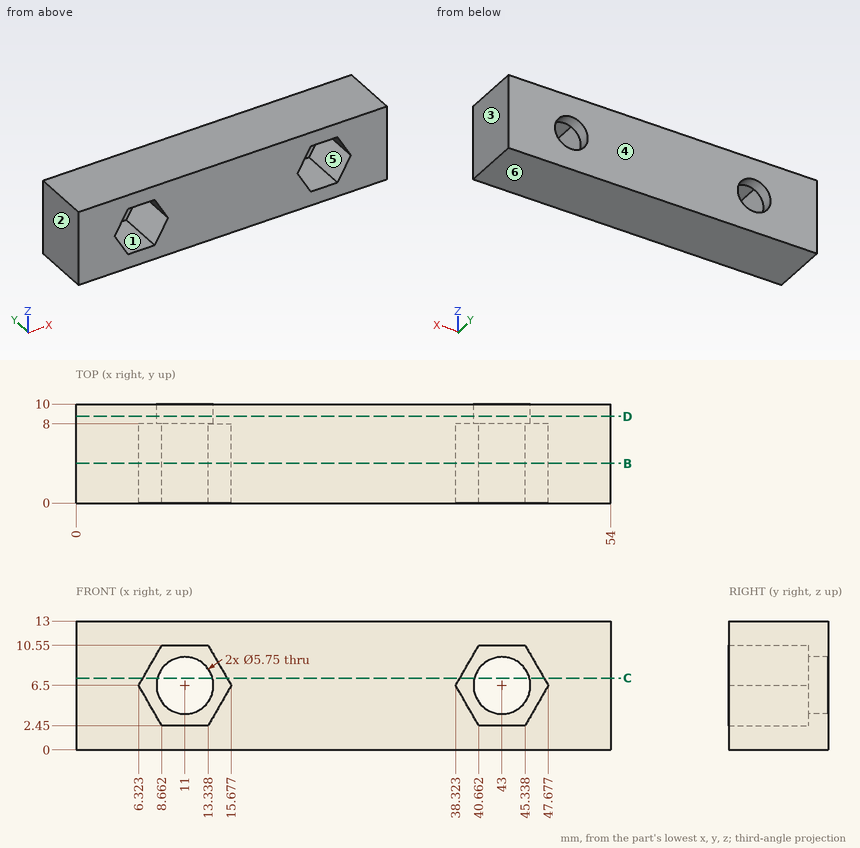
Can you work these out from the drawing? Everything is in mm from the part's minimum corner. A direction names the side the tool comes from. Give positions to 0.01 mm unless a question says otherwise; leave off trailing zeros. Write each loop counter-clockwise with the first axis right and the second up, starting at its lowest first coordinate (ties: lowest second). Pieces come first, ordered by that corner, then holes. Notation, with made-up numbers: M 46.5,6 L 85.5,6 A18 cw 85.5,12 Z; hole C 58.25,-21 d3. An arc over 180 degrees is marked long. Answer in a Markdown table with one row per item. Add a question column.
Item 1: Imagine slicing it at C-C, the plane z = 7.25. Write out the boundary of the cut face in (x, y) (1 decimal), plus the area to 3 significant figures.
Item 2: Imagine slicing it at B-B, the plane y = 4. Write out the boundary of the cut face in (x, z).
Item 3: We'd pull the mould along X, two halves only. Please class the marked faces 1, 2, 3 and 4: released by +X, released by -X, zero draft, split by the parting line, or undercut.
Item 4: Please list where these lines run through material, in increasing order: L1, parallel to Z at x = 43, y = 9.35 (1 decimal); L2, parallel to X at y = 4, z = 7.5; L3, parallel to X at y = 1, z = 6.75.
Item 5: Imagine slicing it at D-D, the plane y = 8.75. State how many separate pieces and enclosed holes the cut face has, plus the area to 3 significant figures.
Item 6: On a 3-axis mill with a long thin cutter (end or side, diameter ignored), from which of +Z, -Z, +X, -X, +Y, -Y can I reach the whole of each face in a straight line? I mean the marked faces 5 and 6. Say none if no direction works.
Item 7: For pin 1 Ø4 at (x, z) = (42, 8) entering from -Y; pin 2 Ø3.5 at (x, z) = (43, 6.5) entering from -Y, each with a flat end and sliding along its axis, tell me the tip position at first contact or that it passes through.
Evaluation:
| question | item | result |
|---|---|---|
| 1 | outline | M 0,0 L 6.8,0 L 6.8,8 L 8.2,8 L 8.2,10 L 0,10 Z; M 13.8,8 L 15.2,8 L 15.2,0 L 38.8,0 L 38.8,8 L 40.2,8 L 40.2,10 L 13.8,10 Z; M 45.8,8 L 47.2,8 L 47.2,0 L 54,0 L 54,10 L 45.8,10 Z |
| 1 | area | 382 mm² |
| 2 | outline | M 0,0 L 54,0 L 54,13 L 0,13 Z; hole M 6.32,6.5 L 8.66,2.45 L 13.34,2.45 L 15.68,6.5 L 13.34,10.55 L 8.66,10.55 Z; hole M 38.32,6.5 L 40.66,2.45 L 45.34,2.45 L 47.68,6.5 L 45.34,10.55 L 40.66,10.55 Z |
| 3 | face 1 | undercut |
| 3 | face 2 | released by -X |
| 3 | face 3 | released by +X |
| 3 | face 4 | zero draft |
| 4 | L1 | z = 0 to 3.6, 9.4 to 13 |
| 4 | L2 | x = 0 to 6.9, 15.1 to 38.9, 47.1 to 54 |
| 4 | L3 | x = 0 to 6.47, 15.53 to 38.47, 47.53 to 54 |
| 5 | separate pieces | 1 |
| 5 | enclosed holes | 2 |
| 5 | area | 650 mm² |
| 6 | face 5 | -Y |
| 6 | face 6 | -Z, +X, -X, +Y, -Y |
| 7 | pin 1 | stops at y = 8 |
| 7 | pin 2 | passes through |
